Read the model definition and answer for the solid it produces. Units are mm, in the model's axes. Face numbers are marked on the shaded views. Coordinates: 2 decimals unless noted, no trailing zeros. Order: outer loops, then holes, each group sorted by start corner. A loop starts at its lowest first (then second) coordinate and runs counter-clockwise, first axis right, second up. Notation, with made-up numbers: M -13.75,21.25 L 11.25,21.25 A33 cw 11.25,55.25 Z; hole C 35.5,54.25 d9. An arc over 180 degrees is marked long. Put each result on its own line as item: value.
from build123d import *

# Parameters (mm, degrees)
SKETCH1_R           = 6.5
BOSS_EXTRUDE1_DEPTH = 14
SKETCH2_R           = 3.2
CUT_EXTRUDE1_DEPTH  = 17.748134224
SKETCH3_R           = 6.5
SKETCH3_R_2         = 6
CUT_EXTRUDE2_DEPTH  = 7
SKETCH4_R           = 1.5
CUT_EXTRUDE3_DEPTH  = 7


with BuildPart() as part:
    # Sketch1 → Boss-Extrude1 (new body)
    with BuildSketch(Plane.XY):
        Circle(SKETCH1_R)
    extrude(amount=BOSS_EXTRUDE1_DEPTH)

    # Sketch2 → Cut-Extrude1 (cut, through all)
    with BuildSketch(Plane.XY.offset(14)):
        Circle(SKETCH2_R)
    extrude(amount=-CUT_EXTRUDE1_DEPTH, mode=Mode.SUBTRACT)

    # Sketch3 → Cut-Extrude2 (cut)
    with BuildSketch(Plane(origin=(0, 0, 1), x_dir=(-1, 0, 0), z_dir=(0, 0, -1))):
        Circle(SKETCH3_R)
        Circle(SKETCH3_R_2, mode=Mode.SUBTRACT)
    extrude(amount=-CUT_EXTRUDE2_DEPTH, mode=Mode.SUBTRACT)

    # Sketch4 → Cut-Extrude3 (cut)
    with BuildSketch(Plane(origin=(0, 0, 0), x_dir=(1, 0, 0), z_dir=(0, 1, 0))):
        with Locations(Location((0, -11, 0), (0, 0, 270))):
            Circle(SKETCH4_R)
    extrude(amount=-CUT_EXTRUDE3_DEPTH, mode=Mode.SUBTRACT)


solid = part.part
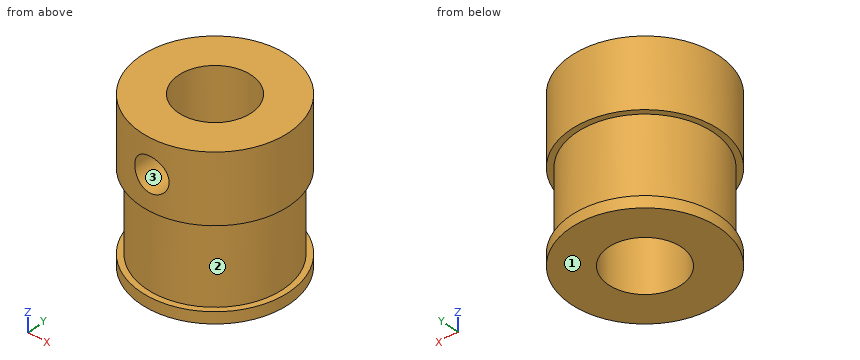
Q1. For a pull along X with two mould halves and no side action, classify the marked faces 1, 2 and 3 as +X half, -X half, draft (parallel to the pull), parting line (faces both ways), or undercut.
Answers below:
face 1: draft
face 2: parting line
face 3: undercut
Q2. Consider line 1 along Y through (x, z) = (0, 3.75); line 2 along Z through (x, y) = (0, -4.25); line 3 along Z through (x, y) = (6, -1.75). Determine where each line is inside the solid, lowest interval first.
Answers below:
line 1: y = -6 to -3.2, 3.2 to 6
line 2: z = 0 to 9.5, 12.5 to 14
line 3: z = 0 to 1, 8 to 14
Q3. Find section C-C on y = -4. Write down the section's boundary in (x, z).
Answers below:
outline: M -5.12,0 L 5.12,0 L 5.12,1 L 4.47,1 L 4.47,8 L 5.12,8 L 5.12,14 L -5.12,14 L -5.12,8 L -4.47,8 L -4.47,1 L -5.12,1 Z; hole C 0,11 d3
Q4. Given pin 1 (6 mm diameter, centred on x = 1.5, z = 4.5, fed in from +Y), flat-ended and moving along its own axis, determine where the tip first touches the part or whether it passes through.
Answers below:
pin 1: stops at y = 6
Q5. Find section A-A on y = 0. Write down the section's boundary in (x, z).
Answers below:
outline: M -6.5,0 L -3.2,0 L -3.2,14 L -6.5,14 L -6.5,8 L -6,8 L -6,1 L -6.5,1 Z; M 3.2,0 L 6.5,0 L 6.5,1 L 6,1 L 6,8 L 6.5,8 L 6.5,14 L 3.2,14 Z
Q6. Find section B-B on x = 0. Write down the section's boundary in (y, z), plus the area to 3 significant figures.
Answers below:
outline: M -6.5,0 L -3.2,0 L -3.2,9.5 L -6.5,9.5 L -6.5,8 L -6,8 L -6,1 L -6.5,1 Z; M -6.5,12.5 L -3.2,12.5 L -3.2,14 L -6.5,14 Z; M 3.2,0 L 6.5,0 L 6.5,1 L 6,1 L 6,8 L 6.5,8 L 6.5,14 L 3.2,14 Z
area: 75.5 mm^2
Q7. Find section D-D on z = 9.25. Write down the section's boundary in (x, y), plus the area to 3 significant figures.
Answers below:
outline: C 0,0 d13; hole C 0,0 d6.4
area: 101 mm^2
